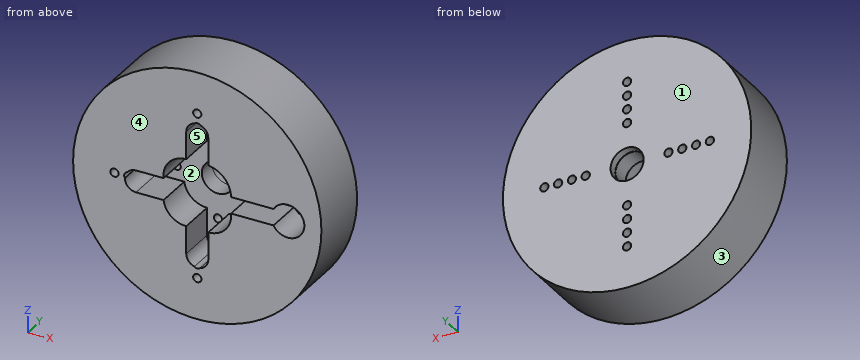
Solid Edge part; units mm, degrees
sketch "Sketch1" plane through (0, 0, 0) normal (0, -1, 0) x (1, 0, 0)
  circle A0 centre (80.5127, 55.3877) radius 22.5
extrude "Protrusion1" add sketch "Sketch1" against normal blind 10
sketch "Sketch2" plane through (80.5127, 10, 55.3877) normal (0, 1, 0) x (0, 0, -1)
  circle A0 centre (0, 0) radius 2.95
extrude "ExtrudedCutout_5" cut sketch "Sketch2" against normal blind 4
sketch "Sketch3" plane through (80.5127, 6, 55.3877) normal (0, 1, 0) x (-1, 0, 0)
  circle A0 centre (0, 0) radius 1.05
extrude "Cutout1" cut sketch "Sketch3" against normal up to next
sketch "Sketch4" plane through (80.5127, 5, 51.1598) normal (0, -1, 0) x (1, 0, 0)
  circle A0 centre (0, 4.2279) radius 3.55
extrude "ExtrudedCutout_7" cut sketch "Sketch4" against normal blind 0.5
chamfer "Chamfer_2" distance 1.9 distance2 0.5 1 edges at (80.5127, 6, 58.3377) measured on face at (78.605, 6, 53.362)
sketch "Sketch5" plane through (80.5127, 10, 55.3877) normal (0, 1, 0) x (0, 0, 1)
  circle A0 centre (0, 0) radius 22.5
  circle A1 centre (0, 0) radius 3
extrude "ExtrudedProtrusion_4" add sketch "Sketch5" along normal blind 1.5
sketch "Sketch6" plane through (80.5127, 0, 55.3877) normal (0, -1, 0) x (0, 0, 1)
  line L0 (1.5, 11.11) -> (1.5, 6.11)
  arc A0 (6.11, 2) -> (1.5, 6.11) centre (1.9729, 2) ccw
  line L1 (6.11, 2) -> (11.11, 2)
  arc A1 (11.11, 2) -> (11.11, -2) centre (11.11, 0) cw
  line L2 (11.11, -2) -> (6.11, -2)
  arc A2 (1.4978, -6.11) -> (6.11, -2) centre (1.4978, -1.4671) ccw
  line L3 (1.4978, -13.81) -> (1.4978, -6.11)
  arc A3 (-1.5, -13.81) -> (1.4978, -13.81) centre (-0.0011, -16.4087) ccw
  line L4 (-1.5, -6.11) -> (-1.5, -13.81)
  arc A4 (-6.11, -2) -> (-1.5, -6.11) centre (-1.9729, -2) ccw
  line L5 (-11.11, -2) -> (-6.11, -2)
  arc A5 (-11.11, 2) -> (-11.11, -2) centre (-11.11, 0) ccw
  line L6 (-6.11, 2) -> (-11.11, 2)
  arc A6 (-6.11, 2) -> (-2.5, 6.11) centre (-1.9654, 2) cw
  line L7 (-2.5, 11.11) -> (-2.5, 6.11)
  arc A7 (1.5, 11.11) -> (-2.5, 11.11) centre (-0.5, 11.11) ccw
  dimension "D1" = 1.5
  dimension "D2" = 2.5
  dimension "D3" = 6.11
  dimension "D4" = 11.11
  dimension "D5" = 6.11
  dimension "D6" = 1.5
  dimension "D7" = 1.4978
  dimension "D8" = 11.11
extrude "ExtrudedCutout_9" cut sketch "Sketch6" against normal blind 6.7
sketch "Sketch7" plane through (80.5127, 11.5, 55.3877) normal (0, 1, 0) x (0, 0, -1)
  circle A0 centre (7.5, 0) radius 0.75
  circle A1 centre (10, 0) radius 0.75
  circle A2 centre (12.5, 0) radius 0.75
  circle A3 centre (15, 0) radius 0.75
  circle A4 centre (-15, 0) radius 0.75
  circle A5 centre (-12.5, 0) radius 0.75
  circle A6 centre (-10, 0) radius 0.75
  circle A7 centre (-7.5, 0) radius 0.75
  circle A8 centre (0, -10) radius 0.75
  circle A9 centre (0, -12.5) radius 0.75
  circle A10 centre (0, -15) radius 0.75
  circle A11 centre (0, -7.5) radius 0.75
  circle A12 centre (0, 7.5) radius 0.75
  circle A13 centre (0, 10) radius 0.75
  circle A14 centre (0, 12.5) radius 0.75
  circle A15 centre (0, 15) radius 0.75
extrude "Cutout2" cut sketch "Sketch7" against normal through all
The listing builds one solid part. Answer for the finished solid, in the listing's coordinates (mm). Face numbers are marked on the shaded views. A direction names the side the tool comes from. Give positions to 0.01 mm unless a question says otherwise; leave off trailing zeros. Loops run counter-clockwise (first coordinate to the right, second up) from the corner with the lowest first, then second, coordinate; pieces in that order, holes last. Notation, with made-up numbers: (-33, -6) - (6, -6) arc R27 ccw to (6, 21) - close; hole circle Ø3 at (-28, -27.5). An arc over 180 degrees is marked (long way). Answer as CSV lines item,"result". Start each with the question number.
Item 1: Find the intervals of material crossed by line 1 (Z direction, x = 98, y = 6); line 2 (Z direction, x = 69, y = 1.25); line 3 (X direction, y = 9.5, z = 41), in increasing order. Write a range as from..to.
Item 2: For the marked faces 4 and 5, determine the directions among +Z, -Z, +X, -X, +Y, -Y from which every point of the face is accessible in a straight line to the end or side of a thin tool.
Item 3: Each of these flat-tipped pins is pushed along its axis until it touches: pin 1 (5.5 mm diameter, centred on x = 71.5, y = 3, fed in from -Z); pin 2 (6 mm diameter, centred on x = 65.5, y = 9, fed in from -Z); pin 3 (5 mm diameter, centred on x = 72, z = 71.5, fed in from -Y); pin 4 (5.5 mm diameter, centred on y = 3.5, z = 64.5, fed in from -X). Where does it stop, or does it pass through?
Item 4: A cutting plane is placed at C-C on z = 74. Determine the outline of the cut face in (x, y), then the cut area to 3 significant figures.
Item 5: A cutting plane is placed at B-B on y = 6. Determine the outline of the cut face in (x, z), then the cut area to 3 significant figures.
Item 6: A cutting plane is placed at A-A on z = 57.5. Determine the outline of the cut face in (x, y).
Item 7: The mould has two halves that part along X. Classify the marked faces 1, 2 and 3: +X half, -X half, draft (parallel to the pull), parting line (faces both ways), or undercut.
Found:
1,line 1,"z = 41.23..52.59, 58.19..69.55"
1,line 2,"z = 36.06..52.93, 56.85..74.72"
1,line 3,"x = 63.21..80.08, 80.95..97.81"
2,face 4,"+Z, -Z, +X, -X, -Y"
2,face 5,"-Y"
3,pin 1,"stops at z = 33.78"
3,pin 2,"stops at z = 36.36"
3,pin 3,"stops at y = 0"
3,pin 4,"stops at x = 58.93"
4,outline,"(67.87, 0) - (93.16, 0) - (93.16, 11.5) - (67.87, 11.5) - close"
4,area,"291 mm^2"
5,outline,"circle Ø45 at (80.51, 55.39); hole circle Ø1.5 at (65.51, 55.39); hole (67.4, 54.95) arc R2 ccw to (69.4, 52.89) - (74.4, 52.89) arc R4.14 ccw to (78.51, 49.28) - (78.51, 44.28) arc R2 ccw to (79.99, 42.35) arc R0.75 ccw to (81.03, 42.35) arc R2 ccw to (82.51, 44.28) - (82.51, 49.28) arc R4.14 ccw to (86.62, 53.89) - (94.32, 53.89) arc R3 ccw (long way) to (94.32, 56.89) - (86.62, 56.89) arc R4.64 ccw to (82.51, 61.5) - (82.51, 66.5) arc R2 ccw to (81.03, 68.43) arc R0.75 ccw to (79.99, 68.43) arc R2 ccw to (78.51, 66.5) - (78.51, 61.5) arc R4.14 ccw to (74.4, 56.89) - (69.4, 56.89) arc R2 ccw to (67.82, 56.11) arc R0.75 ccw to start; hole circle Ø1.5 at (80.51, 40.39); hole circle Ø1.5 at (80.51, 70.39)"
5,area,"1,320 mm^2"
6,outline,"(58.11, 0) - (74.38, 0) - (74.38, 6.7) - (78.45, 6.7) - (78.45, 10) - (78.38, 10) - (78.38, 11.5) - (58.11, 11.5) - close; (82.57, 6.7) - (86.58, 6.7) - (86.58, 0) - (94.79, 0) - (94.79, 6.7) - (99.05, 6.7) - (99.05, 0) - (102.91, 0) - (102.91, 11.5) - (82.64, 11.5) - (82.64, 10) - (82.57, 10) - close"
7,face 1,"draft"
7,face 2,"undercut"
7,face 3,"parting line"
